Check sheet for the modelled part. Datum: model origin and axes. Units: mm. A direction names the side the tool comes from. Round coordinates to 2 decimals unless told otherwise and drop trailing zeros. Write each loop counter-clockwise with the first axis right and the second up, starting at its lowest first coordinate (ties: lowest second). Pieces come first, ordered by that corner, then holes. Notation, with made-up numbers: (-29, 1.5) - (15, 1.5) arc R21 ccw to (15, 20.5) - close; hole circle Ø4 at (-13, -11.75). An arc over 180 degrees is marked (long way). Answer as a JSON object with one key per item and string values. Group by question number.
Item 1: Sectioned sample at C-C on z = 14.5. Record the boundary of the cut face in (x, y).
Item 2: Sectioned sample at A-A on z = 29.5. Record the boundary of the cut face in (x, y).
Item 3: Release check for a two-part mould opening along X. For faces 6 (the cylindrical face through (30, -15, 44)), 7 (the flat face through (5, -15, 0)), 8 (the flat face through (10, -15, 4)) record: pulls with the +X half, pulls with the -X half, needs draft (parallel to the pull), parting line crosses it, or undercut.
Item 4: Thickness scan on line 1 (X direction, y = -28, z = 37); line 2 (Z direction, x = -82, y = -15); line 3 (Z direction, x = -51.5, y = -2.5). Record the ranges inside material, lowest first.
Item 5: Set-up check for faces 1 (the cylindrical face through (52.5, -14.8, 52)), 2 (the cylindrical face through (9.14, -15.21, 49.1)), 3 (the flat face through (10, -20.5, 46.5)), 4 (the flat face through (-78, -15, 35)), 5 (the flat face through (-37, -15, 50)): record each of +Z, -Z, +X, -X, +Y, -Y from which the full face is reachable in a straight line by a thin tool's end or side.
Item 6: Sectioned sample at B-B on x = -39.5. Record the boundary of the cut face in (y, z).
Item 7: Gauge pin test, flat ends, axial feed: P1, Ø1, axis at x = -21, y = -17, coming from the +Z side; P2, Ø15, axis at x = -35.5, y = -10, coming from the -Z side; P3, Ø4.5, axis at x = 38, y = -14.5, coming from the -Z side. Record the tip position at first contact, or that the pin passes through.
```python
from build123d import *

# Parameters (mm, degrees)
F1_DEPTH = 30
F2_R     = 1
F3_DEPTH = 10
F5_DEPTH = 40
F7_DEPTH = 5
F8_R     = 20
F9_R     = 2.99999
F10_R    = 2
F11_R    = 10
F12_R    = 5


# Not quite as in the source:
# - a fillet or chamfer is up to 0.001 mm smaller than in the source, because OpenCascade refuses the exact size


with BuildPart() as f1:
    # F0 (on Front) → F1 (new body)
    with BuildSketch(Plane.XZ):
        Polygon((0, 45), (0, 0), (10, 0), (10, 50), (-88, 50), (-88, 25), (-78, 25), (-78, 45), align=None)
    extrude(amount=F1_DEPTH)

    # F2 (on face) → F3 (cut, through all)
    with BuildSketch(Plane(origin=(-88, 0, 0), x_dir=(0, -1, 0), z_dir=(-1, 0, 0))):
        with Locations((15, 37.5)):
            Circle(F2_R)
    extrude(amount=-F3_DEPTH, mode=Mode.SUBTRACT)

    # F4 (on face) → F5 (join)
    with BuildSketch(Plane.YZ.offset(10)):
        with BuildLine():
            Line((0, 27.2287565553), (0, 37.2287565553))
            ThreePointArc((0, 37.2287565553), (-15, 44), (-30, 37.2287565553))
            Line((-30, 37.2287565553), (-30, 27.2287565553))
            Line((-30, 27.2287565553), (0, 27.2287565553))
        make_face()
    extrude(amount=F5_DEPTH)

    # F6 (on face) → F7 (join)
    with BuildSketch(Plane.YZ.offset(50)):
        with BuildLine():
            Line((0, 37.2287565553), (0, 47.6431808351))
            ThreePointArc((0, 47.6431808351), (-15, 52), (-30, 47.6431808351))
            Line((-30, 47.6431808351), (-30, 37.2287565553))
            ThreePointArc((-30, 37.2287565553), (-15, 44), (0, 37.2287565553))
        make_face()
        with BuildLine():
            Line((0, 27.2287565553), (0, 37.2287565553))
            ThreePointArc((0, 37.2287565553), (-15, 44), (-30, 37.2287565553))
            Line((-30, 37.2287565553), (-30, 27.2287565553))
            Line((-30, 27.2287565553), (0, 27.2287565553))
        make_face()
    extrude(amount=F7_DEPTH)

    # F8
    f8_edges = [f1.edges().sort_by_distance(p)[0] for p in [
        (10, -15, 27.228757),
    ]]
    fillet(f8_edges, radius=F8_R)

    # F9 (radius 3 in the source; OpenCascade refuses exactly that, so slightly less here)
    f9_edges = [f1.edges().sort_by_distance(p)[0] for p in [
        (10, -15, 44),
        (10, -15, 50),
    ]]
    fillet(f9_edges, radius=F9_R)

    # F10
    f10_edges = [f1.edges().sort_by_distance(p)[0] for p in [
        (50, -15, 44),
        (50, -15, 52),
        (55, -15, 52),
    ]]
    fillet(f10_edges, radius=F10_R)

    # F11
    f11_edges = [f1.edges().sort_by_distance(p)[0] for p in [
        (55, -15, 27.228757),
    ]]
    fillet(f11_edges, radius=F11_R)

    # F12
    f12_edges = [f1.edges().sort_by_distance(p)[0] for p in [
        (-88, -15, 50),
    ]]
    fillet(f12_edges, radius=F12_R)


solid = f1.part
```
Completed:
{
 "1": {"outline": "(0, -30) - (11.37, -30) - (11.37, 0) - (0, 0) - close"},
 "2": {"outline": "(-88, -30) - (-78, -30) - (-78, 0) - (-88, 0) - close; (0, -30) - (51.35, -30) - (51.35, 0) - (0, 0) - close"},
 "3": {"face 6": "undercut", "face 7": "needs draft", "face 8": "pulls with the +X half"},
 "4": {"line 1": "-88 to -78, 0 to 55", "line 2": "25 to 36.5, 38.5 to 50", "line 3": "45 to 50"},
 "5": {"face 1": "+Z, +X", "face 2": "+Z, +Y, -Y", "face 3": "+Z", "face 4": "-Z, +Y, -Y", "face 5": "+Z, -X, +Y, -Y"},
 "6": {"outline": "(-30, 45) - (0, 45) - (0, 50) - (-30, 50) - close"},
 "7": {"P1": "z = 50", "P2": "z = 45", "P3": "z = 27.23"}
}
